For this review, take the finished solid that the model builds, in its own axes (mm). A direction names the side the tool comes from. Round coordinates to 2 decimals unless told otherwise and drop trailing zeros. Write each loop counter-clockwise with the first axis right and the second up, starting at its lowest first coordinate (ties: lowest second). Pieces come first, ordered by that corner, then holes. Notation, with made-up numbers: (-35.5, 54.25) - (13.5, 54.25) arc R5 ccw to (13.5, 61.25) - close; hole circle Ø5 at (82, 25). An arc over 180 degrees is marked (long way). One line per item, written item: value. Start each with the question number.
Q1. Clearance check with flat-ended pins moving along their axes: pin 1 Ø4.5 at (x, y) = (-365.5, 5.5) entering from -Z; pin 2 Ø8 at (y, z) = (-2.5, 228) entering from +X (3 decimals); pin 3 Ø5 at (x, z) = (-57.5, 162.5) entering from -Y. State where each tip first meets the part, or that it passes through.
Q2. Mouldability with a two-part tool opening along X and no side actions: class faces 1 (the face through (-278, 12, 49)), 2 (the face through (-320.21, 6.11, 62.65)) as +X half, -X half, draft (parallel to the pull), parting line (faces both ways), or undercut.
Q3. For probe 1 along X at (y, z) = (8, 175.5); probe 2 along Z at (x, y) = (-107, -4.75); probe 3 along Y at (x, z) = (-337, 284.5), list the stretches that pass through material, from the lowest coordinate up.
Q4. Add section B-B on x = -247.5. Write out the cut boundary in (y, z).
Q5. Tool access review of faces 3 (the face through (-328, 11.485, 39)), 4 (the face through (-142, -8, 22.42)), 5 (the face through (-186, 3, 276)), 6 (the face through (-320, 8, 65)): name each direction out of +Z, -Z, +X, -X, +Y, -Y from which nothing blocks a thin tool from reaching the whole face with its end or side.
Q6. Add section A-A on z = 449.5. Write out the cut boundary in (x, y), and give its area (3 significant figures).
Q7. Add section C-C on y = -8.5. Write out the cut boundary in (x, z).
```python
from build123d import *

# Parameters (mm, degrees)
SM_BASE_FLANGE_1_DEPTH           = 3
SM_EDGE_FLANGE_1_STRIP_W         = 13.48
SM_EDGE_FLANGE_1_STRIP_H         = 3
SM_EDGE_FLANGE_1_STRIP_CUT_DEPTH = 466.526743508
SM_EDGE_FLANGE_1_DEPTH           = 466.526743508
SM_EDGE_FLANGE_2_STRIP_W         = 13.48
SM_EDGE_FLANGE_2_STRIP_H         = 3
SM_EDGE_FLANGE_2_STRIP_CUT_DEPTH = 514.106826818
SM_EDGE_FLANGE_2_DEPTH           = 514.106826818
SM_START                         = -362.76
SM_EDGE_FLANGE_5_DEPTH           = 86.26
SM_START_2                       = -361.26
SM_EDGE_FLANGE_5_2_DEPTH         = 83.26
SM_START_3                       = -1
SM_EDGE_FLANGE_5_3_DEPTH         = 4.216740982
SM_EDGE_FLANGE_6_STRIP_CUT_DEPTH = 83.26
SM_EDGE_FLANGE_6_DEPTH           = 83.26
SM_START_4                       = 3
SM_EDGE_FLANGE_6_PROFILE_W       = 99
SM_EDGE_FLANGE_6_PROFILE_H       = 34.545643213
SM_EDGE_FLANGE_6_FLAT_DEPTH      = 3
SM_START_5                       = -3.74
SM_EDGE_FLANGE_7_DEPTH           = 4.74
SM_START_6                       = -276
SM_EDGE_FLANGE_7_2_DEPTH         = 272.26
SM_EDGE_FLANGE_7_3_DEPTH         = 272.26
SKETCH_29_R                      = 3.25
CUT_EXTRUDE_1_DEPTH              = 5


with BuildPart() as part:
    # Базовая кромка1: sheet metal written as solids
    # Sketch 1 → Базовая кромка1 (new body)
    with BuildSketch(Plane(origin=(0, 0, 0), x_dir=(1, 0, 0), z_dir=(0, 1, 0))):
        Polygon((-367, -536.526743508), (0, -536.526743508), (0, -22.41991669), (-276, -22.41991669), (-276, -70), (-367, -70), align=None)
    extrude(amount=SM_BASE_FLANGE_1_DEPTH)

    # Ребро-кромка1: sheet metal written as solids
    # Ребро-кромка1 strip (on a plane across the edge) → Ребро-кромка1 strip cut (cut)
    with BuildSketch(Plane(origin=(-367, 3, 70), x_dir=(1, 0, 0), z_dir=(0, 0, 1))):
        with Locations((-3, -1.5)):
            Rectangle(SM_EDGE_FLANGE_1_STRIP_W, SM_EDGE_FLANGE_1_STRIP_H)
    extrude(amount=SM_EDGE_FLANGE_1_STRIP_CUT_DEPTH, mode=Mode.SUBTRACT)

    # Ребро-кромка1 section (on a plane across the edge) → Ребро-кромка1 (add)
    with BuildSketch(Plane(origin=(-367, 3, 70), x_dir=(1, 0, 0), z_dir=(0, 0, 1))):
        with BuildLine():
            Line((0, 0.74), (0, 6.325908943))
            Line((0, 6.325908943), (3, 6.325908943))
            Line((3, 6.325908943), (3, 0.74))
            ThreePointArc((3, 0.74), (3.216740982, 0.216740982), (3.74, 0))
            Line((3.74, 0), (3.74, -3))
            ThreePointArc((3.74, -3), (1.095420638, -1.904579362), (0, 0.74))
        make_face()
    extrude(amount=SM_EDGE_FLANGE_1_DEPTH)

    # Ребро-кромка2: sheet metal written as solids
    # Ребро-кромка2 strip (on a plane across the edge) → Ребро-кромка2 strip cut (cut)
    with BuildSketch(Plane(origin=(0, 3, 536.526743508), x_dir=(-1, 0, 0), z_dir=(0, 0, -1))):
        with Locations((-3, -1.5)):
            Rectangle(SM_EDGE_FLANGE_2_STRIP_W, SM_EDGE_FLANGE_2_STRIP_H)
    extrude(amount=SM_EDGE_FLANGE_2_STRIP_CUT_DEPTH, mode=Mode.SUBTRACT)

    # Ребро-кромка2 section (on a plane across the edge) → Ребро-кромка2 (add)
    with BuildSketch(Plane(origin=(0, 3, 536.526743508), x_dir=(-1, 0, 0), z_dir=(0, 0, -1))):
        with BuildLine():
            Line((0, 0.74), (0, 6.325908943))
            Line((0, 6.325908943), (3, 6.325908943))
            Line((3, 6.325908943), (3, 0.74))
            ThreePointArc((3, 0.74), (3.216740982, 0.216740982), (3.74, 0))
            Line((3.74, 0), (3.74, -3))
            ThreePointArc((3.74, -3), (1.095420638, -1.904579362), (0, 0.74))
        make_face()
    extrude(amount=SM_EDGE_FLANGE_2_DEPTH)

    # Ребро-кромка5: read off the stored shape, not the designer's step
    # Ребро-кромка5 outline → Ребро-кромка5 (cut)
    with BuildSketch(Plane.YZ.offset(SM_START)):
        with BuildLine():
            Line((0, 70), (0.012581766, 70))
            ThreePointArc((0.012581766, 70), (0.003146765, 70.15312996), (0, 70.306518036))
            Line((0, 70.306518036), (0, 70))
        make_face()
    extrude(amount=SM_EDGE_FLANGE_5_DEPTH, mode=Mode.SUBTRACT)

    # Sm Edge Flange 5 2 outline → Sm Edge Flange 5 2 (add)
    with BuildSketch(Plane.YZ.offset(SM_START_2)):
        with BuildLine():
            ThreePointArc((0.012581766, 70), (0.346296855, 68.73477411), (1.095420638, 67.661938675))
            Line((1.095420638, 67.661938675), (11.485281374, 57.272077939))
            Line((11.485281374, 57.272077939), (13.606601718, 59.393398282))
            Line((13.606601718, 59.393398282), (3.216740982, 69.783259018))
            ThreePointArc((3.216740982, 69.783259018), (3.056329146, 70.023332296), (3, 70.306518036))
            Line((3, 70.306518036), (3, 70))
            Line((3, 70), (0.012581766, 70))
        make_face()
    extrude(amount=SM_EDGE_FLANGE_5_2_DEPTH)

    # Sm Edge Flange 5 3 outline → Sm Edge Flange 5 3 (cut)
    with BuildSketch(Plane(origin=(0, 0, 0), x_dir=(1, 0, 0), z_dir=(0, 1, 0)).offset(SM_START_3)):
        with BuildLine():
            ThreePointArc((-362.76, -71.806518036), (-362.01, -72.556518036), (-361.26, -71.806518036))
            Line((-361.26, -71.806518036), (-361.26, -70))
            Line((-361.26, -70), (-362.76, -70))
            Line((-362.76, -70), (-362.76, -71.806518036))
        make_face()
        with BuildLine():
            Line((-278, -70), (-278, -71.806518036))
            ThreePointArc((-278, -71.806518036), (-277.25, -72.556518036), (-276.5, -71.806518036))
            Line((-276.5, -71.806518036), (-276.5, -70))
            Line((-276.5, -70), (-278, -70))
        make_face()
    extrude(amount=SM_EDGE_FLANGE_5_3_DEPTH, mode=Mode.SUBTRACT)

    # Ребро-кромка6: sheet metal written as solids
    # Ребро-кромка6 strip (on a plane across the edge) → Ребро-кромка6 strip cut (cut)
    with BuildSketch(Plane(origin=(-361.26, 11.485281374, 57.272077939), x_dir=(0, -1, 0), z_dir=(1, 0, 0))):
        Polygon((-11.436378772, 7.193738085), (-1.904579362, -2.338061325), (0.216740982, -0.216740982), (-9.315058428, 9.315058428), align=None)
    extrude(amount=SM_EDGE_FLANGE_6_STRIP_CUT_DEPTH, mode=Mode.SUBTRACT)

    # Ребро-кромка6 bend section (on a plane across the edge) → Ребро-кромка6 (add)
    with BuildSketch(Plane(origin=(-361.26, 11.485281374, 57.272077939), x_dir=(0, -1, 0), z_dir=(1, 0, 0))):
        with BuildLine():
            Line((-3, 0.306518036), (0, 0.306518036))
            ThreePointArc((0, 0.306518036), (0.056329146, 0.023332296), (0.216740982, -0.216740982))
            Line((0.216740982, -0.216740982), (-1.904579362, -2.338061325))
            ThreePointArc((-1.904579362, -2.338061325), (-2.715309452, -1.124718001), (-3, 0.306518036))
        make_face()
    extrude(amount=SM_EDGE_FLANGE_6_DEPTH)

    # Ребро-кромка6 profile (on flange) → Ребро-кромка6 flat (add)
    with BuildSketch(Plane(origin=(0, 11.485281374, 57.272077939), x_dir=(1, 0, 0), z_dir=(0, 1, 0)).offset(SM_START_4)):
        with Locations((-327.5, 17.579339643)):
            Rectangle(SM_EDGE_FLANGE_6_PROFILE_W, SM_EDGE_FLANGE_6_PROFILE_H)
    extrude(amount=-SM_EDGE_FLANGE_6_FLAT_DEPTH)

    # Ребро-кромка7: read off the stored shape, not the designer's step
    # Ребро-кромка7 outline → Ребро-кромка7 (cut)
    with BuildSketch(Plane.YZ.offset(SM_START_5)):
        with BuildLine():
            Line((3.74, 22.41991669), (3.74, 23.15991669))
            Line((3.74, 23.15991669), (0, 23.15991669))
            ThreePointArc((0, 23.15991669), (-0.216740982, 22.636657672), (-0.74, 22.41991669))
            Line((-0.74, 22.41991669), (-15, 22.41991669))
            Line((-15, 22.41991669), (-15, 19.41991669))
            Line((-15, 19.41991669), (-0.74, 19.41991669))
            ThreePointArc((-0.74, 19.41991669), (1.628543857, 20.265508287), (2.926060556, 22.41991669))
            Line((2.926060556, 22.41991669), (3.74, 22.41991669))
        make_face()
    extrude(amount=SM_EDGE_FLANGE_7_DEPTH, mode=Mode.SUBTRACT)

    # Sm Edge Flange 7 2 outline → Sm Edge Flange 7 2 (cut)
    with BuildSketch(Plane.YZ.offset(SM_START_6)):
        with BuildLine():
            Line((2.926060556, 22.41991669), (3.74, 22.41991669))
            Line((3.74, 22.41991669), (3.74, 23.15991669))
            Line((3.74, 23.15991669), (3, 23.15991669))
            ThreePointArc((3, 23.15991669), (2.981469231, 22.788074304), (2.926060556, 22.41991669))
        make_face()
    extrude(amount=SM_EDGE_FLANGE_7_2_DEPTH, mode=Mode.SUBTRACT)

    # Sm Edge Flange 7 3 outline → Sm Edge Flange 7 3 (add)
    with BuildSketch(Plane.YZ.offset(SM_START_6)):
        with BuildLine():
            ThreePointArc((2.926060556, 22.41991669), (2.981469231, 22.788074304), (3, 23.15991669))
            Line((3, 23.15991669), (0, 23.15991669))
            ThreePointArc((0, 23.15991669), (-0.216740982, 22.636657672), (-0.74, 22.41991669))
            Line((-0.74, 22.41991669), (-15, 22.41991669))
            Line((-15, 22.41991669), (-15, 19.41991669))
            Line((-15, 19.41991669), (-0.74, 19.41991669))
            ThreePointArc((-0.74, 19.41991669), (1.628543857, 20.265508287), (2.926060556, 22.41991669))
        make_face()
    extrude(amount=SM_EDGE_FLANGE_7_3_DEPTH)

    # Эскиз29 → Вырез-Вытянуть1 (cut)
    with BuildSketch(Plane(origin=(0, 3, 0), x_dir=(1, 0, 0), z_dir=(0, 1, 0))):
        with Locations(Location((-345.974710107, -153.138626068, 0), (0, 0, 270))):
            Circle(SKETCH_29_R)
        with Locations(Location((-339.843991697, -403.063443347, 0), (0, 0, 270))):
            Circle(SKETCH_29_R)
    extrude(amount=-CUT_EXTRUDE_1_DEPTH, mode=Mode.SUBTRACT)


solid = part.part
```
Result set:
1. pin 1: stops at z = 70
1. pin 2: stops at x = -0.745
1. pin 3: stops at y = 0
2. face 1: undercut
2. face 2: draft
3. probe 1: x = -367 to -364, -3 to 0
3. probe 2: z = 19.42 to 22.42
3. probe 3: y = 0 to 3
4. outline: (-15, 19.42) - (-0.74, 19.42) arc R3.74 ccw to (3, 23.16) - (3, 536.53) - (0, 536.53) - (0, 23.16) arc R0.74 cw to (-0.74, 22.42) - (-15, 22.42) - close
5. face 3: -Z, +X, -X, -Y
5. face 4: +Z, +X, -X, -Y
5. face 5: +Z, +Y
5. face 6: +Z, -X, +Y
6. outline: (-367, 3.74) arc R3.74 ccw to (-363.26, 0) - (-3.74, 0) arc R3.74 ccw to (0, 3.74) - (0, 9.33) - (-3, 9.33) - (-3, 3.74) arc R0.74 cw to (-3.74, 3) - (-363.26, 3) arc R0.74 cw to (-364, 3.74) - (-364, 9.33) - (-367, 9.33) - close
6. area: 1,130 mm^2
7. outline: (-276, 19.42) - (-3.74, 19.42) - (-3.74, 22.42) - (-276, 22.42) - close
